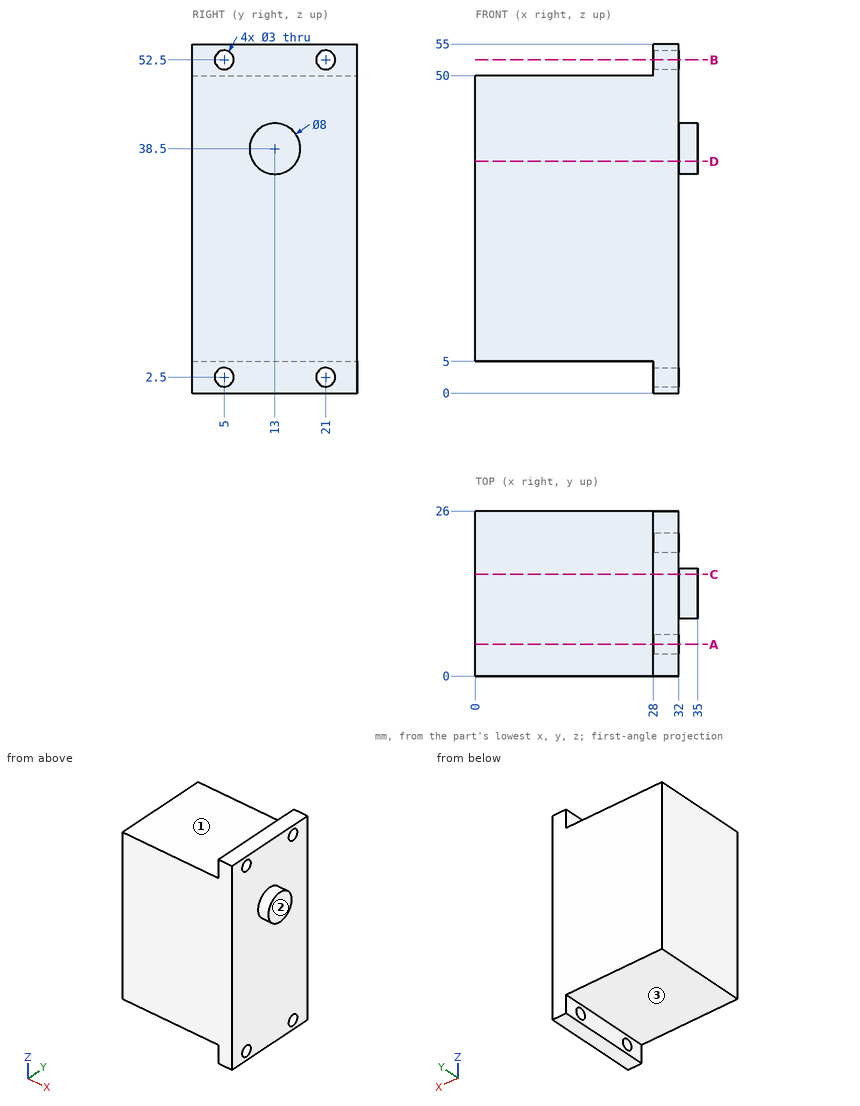
Check sheet for the drawn part. Datum: minimum x, y, z corner. Units: mm. A direction names the side the tool comes from. Give positions to 0.01 mm unless a question says otherwise; leave off trailing zeros. Order: outer loops, then holes, each group sorted by start corner. A loop starts at its lowest first (then second) coordinate and runs counter-clockwise, first axis right, second up. Notation, with made-up numbers: (40.25, -11) -> (47.25, -11) arc R27 ccw to (47.25, 26) -> close; hole circle Ø9 at (89, -9.5). An arc over 180 degrees is marked (long way). One line per item, written item: value.
(1) Tool access check on the marked faces 1, 2 and 3. Record the directions out of +Z, -Z, +X, -X, +Y, -Y that give a thin tool (end or side, any length) a straight path to the whole face; none if there is none.
Final values:
face 1: +Z, -X, +Y, -Y
face 2: +Z, -Z, +X, +Y, -Y
face 3: -Z, -X, +Y, -Y
(2) Sectioned sample at A-A on y = 5. Record the cut outline in (x, z).
Final values:
outline: (0, 5) -> (28, 5) -> (28, 4) -> (32, 4) -> (32, 51) -> (28, 51) -> (28, 50) -> (0, 50) -> close; (28, 0) -> (32, 0) -> (32, 1) -> (28, 1) -> close; (28, 54) -> (32, 54) -> (32, 55) -> (28, 55) -> close
(3) Sectioned sample at C-C on y = 16. Record the cut outline in (x, z), then the cut area to 3 significant figures.
Final values:
outline: (0, 5) -> (28, 5) -> (28, 0) -> (32, 0) -> (32, 35.85) -> (35, 35.85) -> (35, 41.15) -> (32, 41.15) -> (32, 55) -> (28, 55) -> (28, 50) -> (0, 50) -> close
area: 1,500 mm^2
(4) Gauge pin test, flat ends, axial feed: pin 1 (6 mm diameter, centred on y = 6.5, z = 33.5, fed in from -X); pin 2 (3.5 mm diameter, centred on y = 21, z = 52.5, fed in from -X); pin 3 (13 mm diameter, centred on x = 12.5, y = 9.5, fed in from +Z). Record the tip position at first contact, or that the pin passes through.
Final values:
pin 1: x = 0
pin 2: x = 28
pin 3: z = 50
(5) Sectioned sample at B-B on z = 52.5. Record the cut outline in (x, y), then the cut area to 3 significant figures.
Final values:
outline: (28, 0) -> (32, 0) -> (32, 3.5) -> (28, 3.5) -> close; (28, 6.5) -> (32, 6.5) -> (32, 19.5) -> (28, 19.5) -> close; (28, 22.5) -> (32, 22.5) -> (32, 26) -> (28, 26) -> close
area: 80.0 mm^2
(6) Scan lines: line 1 along Z through (x, y) = (30.1, 5); line 2 along Y through (x, z) = (31, 52); line 3 along X through (y, z) = (4.25, 37.5). Record each from-to range of solid material in increasing order. Write a range as [from, to].
Final values:
line 1: [0, 1], [4, 51], [54, 55]
line 2: [0, 3.59], [6.41, 19.59], [22.41, 26]
line 3: [0, 32]
(7) Sectioned sample at D-D on z = 36.5. Record the cut outline in (x, y).
Final values:
outline: (0, 0) -> (32, 0) -> (32, 9.54) -> (35, 9.54) -> (35, 16.46) -> (32, 16.46) -> (32, 26) -> (0, 26) -> close
